Here's how the part is built. I have some questions about the finished solid (model axes, mm). A direction names the side the tool comes from. Give positions to 0.01 mm unless a question says otherwise; leave off trailing zeros. Write each loop counter-clockwise with the first axis right and the second up, starting at its lowest first coordinate (ties: lowest second). Pieces come first, ordered by that corner, then holes. Notation, with made-up numbers: (1.25, -13) -> (38.25, -13) arc R38 cw to (38.25, 26) -> close; hole circle Ø4 at (31, 79). An arc over 180 degrees is marked (long way). Answer as CSV lines item,"result". Start each with the question number.
from build123d import *

# Parameters (mm, degrees)
SKETCH1_R           = 19
BOSS_EXTRUDE1_DEPTH = 2
SKETCH3_W           = 58
SKETCH3_H           = 58
BOSS_EXTRUDE2_DEPTH = 10
SKETCH4_R           = 29
BOSS_EXTRUDE3_DEPTH = 91.5
SKETCH5_R           = 2.5
CUT_EXTRUDE1_DEPTH  = 10
SKETCH6_R           = 3
CUT_EXTRUDE2_DEPTH  = 12
SKETCH7_R           = 1.5
CUT_EXTRUDE4_DEPTH  = 30


with BuildPart() as part:
    # Sketch1 → Boss-Extrude1 (new body)
    with BuildSketch(Plane.XY):
        Circle(SKETCH1_R)
    extrude(amount=-BOSS_EXTRUDE1_DEPTH)

    # Sketch3 → Boss-Extrude2 (add)
    with BuildSketch(Plane(origin=(0, 0, -2), x_dir=(-1, 0, 0), z_dir=(0, 0, -1))):
        Rectangle(SKETCH3_W, SKETCH3_H)
    extrude(amount=BOSS_EXTRUDE2_DEPTH)

    # Sketch4 → Boss-Extrude3 (add)
    with BuildSketch(Plane(origin=(0, 0, -12), x_dir=(-1, 0, 0), z_dir=(0, 0, -1))):
        Circle(SKETCH4_R)
    extrude(amount=BOSS_EXTRUDE3_DEPTH)

    # Sketch5 → Cut-Extrude1 (cut)
    with BuildSketch(Plane.XY.offset(-2)):
        with Locations((-23.5, 23.5)):
            Circle(SKETCH5_R)
        with Locations((23.5, 23.5)):
            Circle(SKETCH5_R)
        with Locations((23.5, -23.5)):
            Circle(SKETCH5_R)
        with Locations((-23.5, -23.5)):
            Circle(SKETCH5_R)
    extrude(amount=-CUT_EXTRUDE1_DEPTH, mode=Mode.SUBTRACT)

    # Sketch6 → Cut-Extrude2 (cut)
    with BuildSketch(Plane.XY):
        Circle(SKETCH6_R)
    extrude(amount=-CUT_EXTRUDE2_DEPTH, mode=Mode.SUBTRACT)

    # Sketch7 → Cut-Extrude4 (cut, through all)
    with BuildSketch(Plane(origin=(0, 0, 0), x_dir=(0, 0, -1), z_dir=(1, 0, 0))):
        with Locations((88.5, 0)):
            Circle(SKETCH7_R)
    extrude(amount=-CUT_EXTRUDE4_DEPTH, mode=Mode.SUBTRACT)


solid = part.part
Item 1: For faces 4 (the face through (-21, -22, -12)), 5 (the face through (22, 21, -12)), 6 (the face through (22, -21, -12)), 7 (the face through (0, 0, -88)), 8 (the face through (8.767, -16.856, -0.986)), which set-ups out of +Z, -Z, +X, -X, +Y, -Y let a thin tool reach every point of the face, with its end or its side?
Item 2: I'm going to push flat-ended pins straight in: pin 1 (12 mm diameter, centred on y = 13.5, z = -21.5, fed in from +X); pin 2 (2 mm diameter, centred on y = 20.5, z = -53.5, fed in from -X); pin 3 (8 mm diameter, centred on x = -23.5, y = -23.5, fed in from +Z). Where does each tip first touch, or does it pass through?
Item 3: If we section it at A-A (x = -24): Please give me the cut outline in (y, z), and give its area (3 significant figures).
Item 4: If we section it at B-B (x = 23.5): Please give me the cut outline in (y, z).
Item 5: We'd pull the mould along Y, two halves only. Please class faces 1 (the face through (0, 0, -103.5)), 2 (the face through (-13.38, -25.73, -57.11)), 3 (the face through (0, 0, -12)): released by +Y, released by -Y, zero draft, split by the parting line, or undercut.
Item 6: If I drill on line 1 (Y direction, x = -23.5, z = -7); line 2 (Y direction, x = -0.5, z = -61.5); line 3 (Z direction, x = -1.5, y = -19.5), over which ranges is the centre line in solid material (lowest first)? Write a range as [from, to].
Final values:
1,face 4,"-Z, -X, -Y"
1,face 5,"-Z, +X, +Y"
1,face 6,"-Z, +X, -Y"
1,face 7,"-X"
1,face 8,"+Z"
2,pin 1,"x = 28.01"
2,pin 2,"x = -21.47"
2,pin 3,"z = -2"
3,outline,"(-29, -12) -> (-25.95, -12) -> (-25.95, -2) -> (-29, -2) -> close; (-21.05, -12) -> (-16.28, -12) -> (-16.28, -103.5) -> (16.28, -103.5) -> (16.28, -12) -> (21.05, -12) -> (21.05, -2) -> (-21.05, -2) -> close; (25.95, -12) -> (29, -12) -> (29, -2) -> (25.95, -2) -> close; hole circle Ø3 at (0, -88.5)"
3,area,"3,450 mm2"
4,outline,"(-29, -12) -> (-26, -12) -> (-26, -2) -> (-29, -2) -> close; (-21, -12) -> (-16.99, -12) -> (-16.99, -103.5) -> (16.99, -103.5) -> (16.99, -12) -> (21, -12) -> (21, -2) -> (-21, -2) -> close; (26, -12) -> (29, -12) -> (29, -2) -> (26, -2) -> close"
5,face 1,"zero draft"
5,face 2,"split by the parting line"
5,face 3,"undercut"
6,line 1,"[-29, -26], [-21, 21], [26, 29]"
6,line 2,"[-29, 29]"
6,line 3,"[-103.5, -2]"
